CAD build for the part. Positions are in the model's coordinates, mm. A direction names the side the tool comes from. Give positions to 0.01 mm unless a question says otherwise; leave off trailing zeros. Loops run counter-clockwise (first coordinate to the right, second up) from the corner with the lowest first, then second, coordinate; pieces in that order, holes last. Notation, with made-up numbers: M 63,55.25 L 114,55.25 A20 cw 114,74.25 Z; hole C 54.25,42 d10. An arc over 180 degrees is marked long. Answer as CSV lines item,"result".
```python
from build123d import *

# Parameters (mm, degrees)
F1_DEPTH = 20
F2_R     = 2.5
F3_DEPTH = 50
F4_R     = 2.99999


# Not quite as in the source:
# - a fillet or chamfer is up to 0.001 mm smaller than in the source, because OpenCascade refuses the exact size


with BuildPart() as f1:
    # F0 (on Top) → F1 (new body)
    with BuildSketch(Plane.XY):
        with BuildLine():
            Line((80, 0), (-20.5, 0))
            Line((-20.5, 0), (0, -20.5))
            Line((0, -20.5), (28, -20.5))
            Line((28, -20.5), (28, -33.5))
            Line((28, -33.5), (0, -33.5))
            Line((0, -33.5), (0, -40))
            Line((0, -40), (38, -40))
            Line((38, -40), (38, -20))
            ThreePointArc((38, -20), (42.3933982822, -9.3933982822), (53, -5))
            Line((53, -5), (80, -5))
            Line((80, -5), (80, 0))
        make_face()
    extrude(amount=F1_DEPTH)

    # F2 (on Front) → F3 (cut)
    with BuildSketch(Plane.XZ):
        with Locations((10, 10)):
            Circle(F2_R)
        with Locations((-5.5, 10)):
            Circle(F2_R)
        with Locations((32.5, 10)):
            Circle(F2_R)
        with Locations((67.5, 10)):
            Circle(F2_R)
    extrude(amount=F3_DEPTH, mode=Mode.SUBTRACT)

    # F4 (radius 3 in the source; OpenCascade refuses exactly that, so slightly less here)
    f4_edges = [f1.edges().sort_by_distance(p)[0] for p in [
        (66.5, -5, 20),
        (19, -40, 20),
        (0, -40, 10),
        (19, -40, 0),
        (66.5, -5, 0),
        (-10.25, -10.25, 20),
        (-10.25, -10.25, 0),
        (80, -5, 10),
        (38, -40, 10),
        (28, -27, 20),
        (28, -27, 0),
    ]]
    fillet(f4_edges, radius=F4_R)


solid = f1.part
```
Q1. Cut at B-B (x = 32.5). Write the cut outline in (y, z), and give its area (3 significant figures).
Solution:
outline,"M -40,3 A3 ccw -37,0 L 0,0 L 0,7.5 L -40,7.5 Z; M -40,12.5 L 0,12.5 L 0,20 L -37,20 A3 ccw -40,17 Z"
area,"596 mm²"
Q2. Mould opens along X. For faces 5 (the cylindrical face through (66.69, -4.1, 0.86)), 6 (the cylindrical face through (9.46, -36.7, 7.56)), 7 (the cylindrical face through (37.1, -39.14, 10.1)) say: released by +X, released by -X, zero draft, split by the parting line, or undercut.
Solution:
face 5,"zero draft"
face 6,"undercut"
face 7,"released by +X"
Q3. Which spindle directions (+Z, -Z, +X, -X, +Y, -Y) get a long thin tool onto all of the face, cutting with end or side? Do faces 1 (the cylindrical face through (28.9, -27.09, 0.86)), 2 (the flat face through (38, -29, 10)), 3 (the flat face through (0, -35, 10)), 4 (the cylindrical face through (28.9, -27.09, 19.14)). Say none if no direction does.
Solution:
face 1,"-Z, -X"
face 2,"+Z, -Z, +X, -Y"
face 3,"+Z, -Z, -X, -Y"
face 4,"+Z, -X"
Q4. Cut at D-D (x = 10). Write the cut outline in (y, z).
Solution:
outline,"M -40,3 A3 ccw -37,0 L -33.5,0 L -33.5,7.5 L -40,7.5 Z; M -40,12.5 L -33.5,12.5 L -33.5,20 L -37,20 A3 ccw -40,17 Z; M -20.5,0 L 0,0 L 0,7.5 L -20.5,7.5 Z; M -20.5,12.5 L 0,12.5 L 0,20 L -20.5,20 Z"
Q5. Cut at C-C (y = -23). Write the cut outline in (x, z), and give its area (3 significant figures).
Solution:
outline,"M 28,3 A3 ccw 31,0 L 35,0 A3 ccw 38,3 L 38,17 A3 ccw 35,20 L 31,20 A3 ccw 28,17 Z; hole C 32.5,10 d5"
area,"173 mm²"
Q6. Pin check, flat tips, straight feed: P1, Ø11, axis at y = -24.5, z = 7.5, coming from the +X side; P2, Ø2, axis at x = -4, z = 2.5, coming from the -Y side; P3, Ø1.5, axis at x = 10, z = 12, coming from the +Y side; P4, Ø3, axis at y = -17, z = 12, coming from the +X side. Stop position of each tip, or through.
Solution:
P1,"stops at x = 38.03"
P2,"stops at y = -17.46"
P3,"stops at y = 0"
P4,"stops at x = 38.69"
Q7. Cut at A-A (z = 10). Give the number of separate pieces and of enclosed holes in the cut face, and give its area (3 significant figures).
Solution:
separate pieces,"6"
enclosed holes,"0"
area,"1,180 mm²"
Q8. Wall check: line 1 (X direction, y = -35, z = 10); line 2 (Y direction, x = 22, z = 14.25); line 3 (X direction, y = -17.5, z = 11). Give the ranges that are in metal, low to high. Write a range as [from, to].
Solution:
line 1,"x = [0, 7.5], [12.5, 30], [35, 38]"
line 2,"y = [-40, -33.5], [-20.5, 0]"
line 3,"x = [-3, 7.71], [12.29, 30.21], [34.79, 38.21]"
